Autodesk Inventor part; units mm, degrees
ref_plane "YZ Plane" through (0, 0, 0) normal (1, 0, 0) x (0, 1, 0)
ref_plane "XZ Plane" through (0, 0, 0) normal (0, 1, 0) x (-1, 0, 0)
ref_plane "XY Plane" through (0, 0, 0) normal (0, 0, 1) x (1, 0, 0)
sketch "Sketch1" plane through (0, 0, 0) normal (0, 0, 1) x (1, 0, 0)
  line L0 (-4, 0) -> (4, 0)
  line L1 (-4, 0) -> (-4, 30)
  line L2 (4, 0) -> (4, 30)
  arc A0 (37.2135, 63.2135) -> (-35.9097, 61.9097) centre (1.5, 15) ccw
  line L3 (4, 30) -> (37.2135, 63.2135)
  line L4 (4, 30) -> (59.6428, 30) construction
  line L5 (-4, 30) -> (-35.9097, 61.9097)
  point P0 (0, 0)
  dimension "d0" = 8
  dimension "d1" = 30
  dimension "d2" = 120
  dimension "d3" = 30
  dimension "d4" = 45
  dimension "d6" = 135
extrude "Extrusion1" add sketch "Sketch1" along normal blind 2
sketch "Sketch2" plane through (0, 0, 2) normal (0, 0, 1) x (1, 0, 0)
  circle A0 centre (0, 4) radius 2.6
  line L0 (-4, 0) -> (4, 0)
  dimension "d23" = 5.2
  dimension "d24" = 4
fillet "Fillet3" radius 2 2 edges at (37.2135, 63.2135, 1) (-35.9097, 61.9097, 1)
fillet "Fillet4" radius 2 2 edges at (4, 0, 1) (-4, 0, 1)
fillet "Fillet5" radius 0.5 10 edges at (-34.8764, 61.8612, 2) (-19.1482, 45.1482, 2) (36.1167, 63.1416, 2) (19.7698, 45.7698, 2) (0.3868, 74.9897, 2) (-34.8764, 61.8612, 0) (-19.1482, 45.1482, 0) (36.1167, 63.1416, 0) (19.7698, 45.7698, 0) (0.3868, 74.9897, 0)
extrude "Extrusion5" cut sketch "Sketch2" against normal blind 2
equation "\"d3\" = d1"
properties part number "Part1#2"
CAD build for the part. Positions are in the model's coordinates, mm. Coordinates: 2 decimals unless noted, no trailing zeros. Write each loop counter-clockwise with the first axis right and the second up, starting at its lowest first coordinate (ties: lowest second). Pieces come first, ordered by that corner, then holes. Notation, with made-up numbers: (70, 74) - (100, 74) arc R34 cw to (100, 112) - close; hole circle Ø9 at (16.5, -35.5). An arc over 180 degrees is marked (long way). Use a Markdown table: item, result. Add a question column.
Item 1: Band-saw the part on A-A, the plane z = 0.95. Give the cut face in (x, y), and give its area (3 significant figures).
Item 2: Mould opens along X. For faces 1 (the face through (-0.338, 6.578, 1.014)), 2 (the face through (-4, 16, 1)), 3 (the face through (0, 54, 0)) say: pulls with the +X half, pulls with the -X half, needs draft (parallel to the pull), parting line crosses it, or undercut.
Item 3: Drill centre lines: L1, parallel to Y at x = 0, z = 0.6; L2, parallel to X at y = 8, z = 1.8; L3, parallel to Y at x = 27.5, z = 0.5. Where is each one in solid material? Low to high. Write a range as from..to.
Item 4: Band-saw the part on C-C, the plane y = 23.5. Give the cut face in (x, z), and give its area (3 significant figures).
Item 5: Flat gauge pins, fed straight in: pin 1 (1 mm diameter, centred on y = 22.5, z = 0.5, fed in from -X); pin 2 (0.6 mm diameter, centred on y = 22.5, z = 1, fed in from +X). Where does each tip first touch, or does it go through?
Item 6: Band-saw the part on B-B, the plane y = 4. Give the cut face in (x, z).
Numbers:
| question | item | result |
|---|---|---|
| 1 | outline | (-34.3, 60.3) - (-4, 30) - (-4, 2) arc R2 ccw to (-2, 0) - (2, 0) arc R2 ccw to (4, 2) - (4, 30) - (35.54, 61.54) arc R2 ccw to (35.25, 64.61) arc R60 ccw to (-34.07, 63.32) arc R2 ccw to start; hole circle Ø5.2 at (0, 4) |
| 1 | area | 2,150 mm2 |
| 2 | face 1 | undercut |
| 2 | face 2 | pulls with the -X half |
| 2 | face 3 | needs draft |
| 3 | L1 | 0..1.4, 6.6..74.98 |
| 3 | L2 | -4..4 |
| 3 | L3 | 53.5..69.07 |
| 4 | outline | (-4, 0) - (4, 0) - (4, 2) - (-4, 2) - close |
| 4 | area | 16.0 mm2 |
| 5 | pin 1 | x = -4 |
| 5 | pin 2 | x = 4 |
| 6 | outline | (-4, 0) - (-2.6, 0) - (-2.6, 2) - (-4, 2) - close; (2.6, 0) - (4, 0) - (4, 2) - (2.6, 2) - close |
